```python
from build123d import *

# Parameters (mm, degrees)
F0_W     = 89.724988
F0_H     = 123.777248
F0_W_2   = 71.94499
F0_H_2   = 105.99725
F1_DEPTH = 64.262
F2_R     = 8.769798
F3_DEPTH = 149.86
F4_W     = 66.31229
F4_H     = 46.081694
F5_DEPTH = 136.906


with BuildPart() as f1:
    # F0 (on Top) → F1 (new body)
    with BuildSketch(Plane.XY):
        Rectangle(F0_W, F0_H)
        Rectangle(F0_W_2, F0_H_2, mode=Mode.SUBTRACT)
    extrude(amount=F1_DEPTH)

    # F2 (on face) → F3 (cut)
    with BuildSketch(Plane.XZ.offset(61.888624)):
        with Locations((0, 31.491935)):
            Circle(F2_R)
    extrude(amount=-F3_DEPTH, mode=Mode.SUBTRACT)

    # F4 (on face) → F5 (cut)
    with BuildSketch(Plane(origin=(-44.862494, 0, 0), x_dir=(0, -1, 0), z_dir=(-1, 0, 0))):
        with Locations((0, 64.262)):
            Rectangle(F4_W, F4_H)
    extrude(amount=-F5_DEPTH, mode=Mode.SUBTRACT)


solid = f1.part
```
Input: part model. Units: mm. Frame: model coordinates. A direction names the side the tool comes from. Round coordinates to 2 decimals unless told otherwise and drop trailing zeros. Write each loop counter-clockwise with the first axis right and the second up, starting at its lowest first coordinate (ties: lowest second). Pieces come first, ordered by that corner, then holes. Notation, with made-up numbers: M 39.5,57 L 66.5,57 A32 cw 66.5,87 Z; hole C 12.25,33 d2. An arc over 180 degrees is marked long. Write each question's results on one line, items separated by ' | '.
Q1. Draft query along X for faces 1 (the face through (40, 0, 41.221)), 2 (the face through (-1.9, -57.51, 22.93)), 3 (the face through (-35.972, -1, 25)), 4 (the face through (44.862, -1, 25)). Return one class per face: released by +X, released by -X, zero draft, split by the parting line, or undercut.
Results:
face 1: zero draft | face 2: undercut | face 3: undercut | face 4: released by +X
Q2. Pin query (flat end, axial travel): P1, Ø10, axis at x = 40, y = 2, coming from the +Z side. Return the tip coordinate at first contact, or that it passes through.
Results:
P1: stops at z = 41.22
Q3. Line query: line 1 along Y through (x, z) = (-26.5, 46); line 2 along Z through (x, y) = (0, 59.5); line 3 along X through (y, z) = (20, 26). Output: solid intervals per line, ascending.
Results:
line 1: y = -61.89 to -53, 53 to 61.89 | line 2: z = 0 to 22.72, 40.26 to 64.26 | line 3: x = -44.86 to -35.97, 35.97 to 44.86
Q4. Section query D-D (z = 29). Return loops of the section in (x, y), and give its area (3 significant figures).
Results:
outline: M -44.86,-61.89 L -8.41,-61.89 L -8.41,-53 L -35.97,-53 L -35.97,53 L -8.41,53 L -8.41,61.89 L -44.86,61.89 Z; M 8.41,-61.89 L 44.86,-61.89 L 44.86,61.89 L 8.41,61.89 L 8.41,53 L 35.97,53 L 35.97,-53 L 8.41,-53 Z | area: 3,180 mm^2
Q5. Section query B-B (y = -43.5). Return loops of the section in (x, z), and give its area (3 significant figures).
Results:
outline: M -44.86,0 L -35.97,0 L -35.97,64.26 L -44.86,64.26 Z; M 35.97,0 L 44.86,0 L 44.86,64.26 L 35.97,64.26 Z | area: 1,140 mm^2
Q6. Section query A-A (x = 0). Return loops of the section in (y, z).
Results:
outline: M -61.89,0 L -53,0 L -53,22.72 L -61.89,22.72 Z; M -61.89,40.26 L -53,40.26 L -53,64.26 L -61.89,64.26 Z; M 53,0 L 61.89,0 L 61.89,22.72 L 53,22.72 Z; M 53,40.26 L 61.89,40.26 L 61.89,64.26 L 53,64.26 Z
Q7. Access query for faces 5 (the face through (-40, -33.156, 53)), 6 (the face through (-8, -52.999, 39)), 7 (the face through (9, 61.889, 32)). Directions: +Z, -Z, +X, -X, +Y, -Y. A direction counts if a zero-diameter tool reaches every point of the face in a straight line with its end or side. Return the directions, or none.
Results:
face 5: +Z, +X, -X | face 6: +Z, -Z | face 7: +Z, -Z, +X, -X, +Y
Q8. Section query C-C (x = 20.5). Return loops of the section in (y, z), and give its area (3 significant figures).
Results:
outline: M -61.89,0 L -53,0 L -53,64.26 L -61.89,64.26 Z; M 53,0 L 61.89,0 L 61.89,64.26 L 53,64.26 Z | area: 1,140 mm^2
